The figure shows three views and two pictorial views of one solid part (mm, origin at its lowest corner). Answer the questions. A direction names the side the tool comes from. Coordinates: 2 decimals unless noted, no trailing zeros. Loops run counter-clockwise (first coordinate to the right, second up) from the corner with the lowest first, then second, coordinate; pieces in that order, holes last. Notation, with made-up numbers: (61, -7.5) -> (84, -7.5) arc R8 cw to (84, 4.5) -> close; hole circle Ø10 at (53, 59). An arc over 180 degrees is marked (long way). Answer as a JSON object with one key per item and string values. Group by question number.
1) Section C-C, the plane x = 9 is taken. Give the vertices of the cut face in (y, z), plus the area to 3 significant figures.
2) Section A-A, the plane z = 7 is taken. Give the vertices of the cut face in (x, y), plus the area to 3 significant figures.
3) Section B-B, the plane y = 10 is taken. Give the vertices of the cut face in (x, z).
4) Which of the six approach directions +Z, -Z, +X, -X, +Y, -Y give full straight-line access (tool end or side, diameter ignored) to the marked faces 1, 2, 3 and 4?
5) Consider probe 1 along Y at (x, z) = (5.5, 7); probe 2 along X at (y, z) = (126.5, 3); probe 3 along Z at (x, y) = (7.25, 36). Determine where each line is inside the solid, lowest interval first. Write a range as [from, to].
6) Flat-ended cylindrical pins translate along their axes: P1, Ø0.9, axis at x = 1, z = 4.5, coming from the +Y side; P2, Ø8, axis at x = 12, y = 57, coming from the +Z side; P3, Ø5, axis at x = 11.5, y = 119.5, coming from the +Z side; P4, Ø5, axis at y = 10, z = 7, coming from the -X side. Find the tip coordinate at first contact, or state that the pin passes through.
7) Determine the mould class of the marked faces 5, 6 and 7 for opening direction Y: released by +Y, released by -Y, zero draft, split by the parting line, or undercut.
8) Section D-D, the plane y = 71.5 is taken. Give the vertices of the cut face in (x, z), plus the area to 3 significant figures.
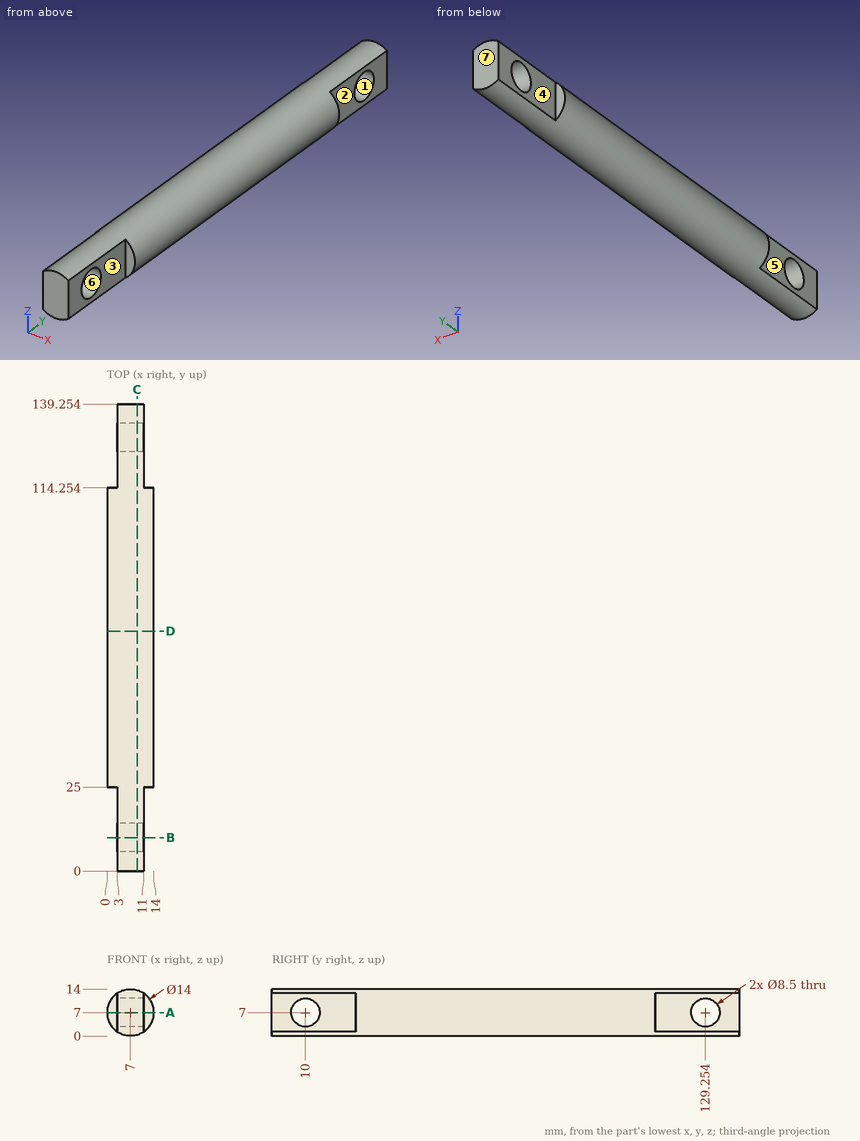
Determined:
{
 "1": {"outline": "(0, 0.29) -> (139.25, 0.29) -> (139.25, 13.71) -> (0, 13.71) -> close; hole circle Ø8.5 at (10, 7); hole circle Ø8.5 at (129.25, 7)", "area": "1,750 mm²"},
 "2": {"outline": "(0, 25) -> (3, 25) -> (3, 14.25) -> (11, 14.25) -> (11, 25) -> (14, 25) -> (14, 114.25) -> (11, 114.25) -> (11, 125) -> (3, 125) -> (3, 114.25) -> (0, 114.25) -> close; (3, 0) -> (11, 0) -> (11, 5.75) -> (3, 5.75) -> close; (3, 133.5) -> (11, 133.5) -> (11, 139.25) -> (3, 139.25) -> close", "area": "1,510 mm²"},
 "3": {"outline": "(3, 1.26) arc R7 ccw to (11, 1.26) -> (11, 2.75) -> (3, 2.75) -> close; (3, 11.25) -> (11, 11.25) -> (11, 12.74) arc R7 ccw to (3, 12.74) -> close"},
 "4": {"face 1": "+X, -X", "face 2": "+Z, -Z, +X, +Y", "face 3": "+Z, -Z, +X, -Y", "face 4": "+Z, -Z, -X, +Y"},
 "5": {"probe 1": "[0, 5.75], [14.25, 125], [133.5, 139.25]", "probe 2": "[3, 11]", "probe 3": "[0, 14]"},
 "6": {"P1": "y = 114.25", "P2": "z = 13.93", "P3": "z = 13.71", "P4": "through"},
 "7": {"face 5": "zero draft", "face 6": "undercut", "face 7": "released by +Y"},
 "8": {"outline": "circle Ø14 at (7, 7)", "area": "154 mm²"}
}
